The listing builds one solid part. Answer for the finished solid, in the listing's coordinates (mm). Coordinates: 2 decimals unless noted, no trailing zeros. Write each loop counter-clockwise with the first axis right and the second up, starting at its lowest first coordinate (ties: lowest second). Pieces come first, ordered by that corner, then holes.
from build123d import *

# Parameters (mm, degrees)
SKETCH1_W           = 55
SKETCH1_H           = 70
SKETCH1_R           = 2
BOSS_EXTRUDE1_DEPTH = 5
SKETCH2_R           = 2.85
CUT_EXTRUDE1_DEPTH  = 8
CHAMFER1_SIZE       = 0.5


with BuildPart() as part:
    # Sketch1 → Boss-Extrude1 (new, symmetric)
    with BuildSketch(Plane(origin=(0, 0, 0), x_dir=(1, 0, 0), z_dir=(0, 1, 0))):
        Rectangle(SKETCH1_W, SKETCH1_H)
        with Locations(Location((18.5, -18.5, 0), (0, 0, 270))):
            Circle(SKETCH1_R, mode=Mode.SUBTRACT)
        with Locations(Location((-18.5, -18.5, 0), (0, 0, 270))):
            Circle(SKETCH1_R, mode=Mode.SUBTRACT)
        with Locations(Location((18.5, 18.5, 0), (0, 0, 270))):
            Circle(SKETCH1_R, mode=Mode.SUBTRACT)
        with Locations(Location((-18.5, 18.5, 0), (0, 0, 270))):
            Circle(SKETCH1_R, mode=Mode.SUBTRACT)
        with BuildLine():
            Line((-10, 27), (10, 27))
            ThreePointArc((10, 27), (12, 29), (10, 31))
            Line((10, 31), (-10, 31))
            ThreePointArc((-10, 31), (-12, 29), (-10, 27))
        make_face(mode=Mode.SUBTRACT)
        with BuildLine():
            Line((-10, -31), (10, -31))
            ThreePointArc((10, -31), (12, -29), (10, -27))
            Line((10, -27), (-10, -27))
            ThreePointArc((-10, -27), (-12, -29), (-10, -31))
        make_face(mode=Mode.SUBTRACT)
    extrude(amount=BOSS_EXTRUDE1_DEPTH, both=True)

    # Sketch2 → Cut-Extrude1 (cut)
    with BuildSketch(Plane(origin=(27.5, 0, 0), x_dir=(0, 0, -1), z_dir=(1, 0, 0))):
        with Locations((-25, 0)):
            Circle(SKETCH2_R)
        with Locations(Location((25, 0, 0), (0, 0, 180))):
            Circle(SKETCH2_R)
    cut_extrude1 = extrude(amount=-CUT_EXTRUDE1_DEPTH, mode=Mode.SUBTRACT)

    # Mirror1: Cut-Extrude1 across plane
    add(cut_extrude1.mirror(Plane(origin=(0, 0, 0), x_dir=(0, 0, 1), z_dir=(1, 0, 0))), mode=Mode.SUBTRACT)

    # Chamfer1
    chamfer1_edges = [part.edges().sort_by_distance(p)[0] for p in [
        (-18.5, 5, 16.5),
        (18.5, 5, -20.5),
        (18.5, 5, 16.5),
        (-18.5, 5, -20.5),
        (27.5, 0, 27.85),
        (27.5, 0, -27.85),
        (-27.5, 0, 27.85),
        (-27.5, 0, -27.85),
    ]]
    chamfer(chamfer1_edges, length=CHAMFER1_SIZE)


solid = part.part
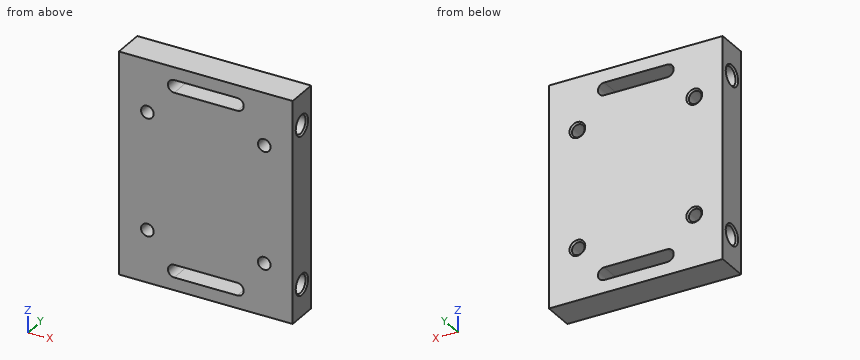
Q1. The part is cut by section D-D, the plane x = 22. Write down the section's boundary in (y, z).
Answers below:
outline: (-5, -35) - (5, -35) - (5, 35) - (-5, 35) - close; hole circle Ø5.7 at (0, -25); hole circle Ø5.7 at (0, 25)
Q2. The part is cut by section A-A, the plane z = -18.5. Write down the section's boundary in (x, y), then the cut area to 4 significant figures.
Answers below:
outline: (-27.5, -5) - (-20.5, -5) - (-20.5, 4.5) - (-21, 5) - (-27.5, 5) - close; (-16.5, -5) - (16.5, -5) - (16.5, 4.5) - (16, 5) - (-16, 5) - (-16.5, 4.5) - close; (20.5, -5) - (27.5, -5) - (27.5, 5) - (21, 5) - (20.5, 4.5) - close
area: 469.5 mm2
Q3. Find the intervals of material crossed by probe 1 along X at (y, z) = (-2.5, 18.5); probe 2 along Z at (x, y) = (6.5, -2.5); probe 3 along Z at (x, y) = (18, 1.5), in increasing order.
Answers below:
probe 1: x = -27.5 to -20.5, -16.5 to 16.5, 20.5 to 27.5
probe 2: z = -35 to -31, -27 to 27, 31 to 35
probe 3: z = -35 to -20.44, -16.56 to 16.56, 20.44 to 35
Q4. The part is cut by section B-B, the plane x = 8.5. Write down the section's boundary in (y, z).
Answers below:
outline: (-5, -35) - (5, -35) - (5, -31) - (-5, -31) - close; (-5, -27) - (5, -27) - (5, 27) - (-5, 27) - close; (-5, 31) - (5, 31) - (5, 35) - (-5, 35) - close
Q5. Given pin 1 (4.5 mm diameter, centred on y = 0, z = 25, fed in from +X); pin 2 (5 mm diameter, centred on y = 0, z = -25, fed in from -X); pin 3 (4.5 mm diameter, centred on x = 18.5, z = 18.5, fed in from +Y), each flat-ended and moving along its own axis, determine where each tip first touches the part or whether it passes through.
Answers below:
pin 1: stops at x = 19.5
pin 2: stops at x = -19.5
pin 3: stops at y = 4.75
Q6. The part is cut by section C-C, the plane z = -30. Write down the section's boundary in (x, y), then the cut area to 3 significant figures.
Answers below:
outline: (-27.5, -5) - (-11.73, -5) - (-11.73, 5) - (-27.5, 5) - close; (11.73, -5) - (27.5, -5) - (27.5, 5) - (11.73, 5) - close
area: 315 mm2
